Model file for the job. Use its own axes, mm. Face numbers are marked on the shaded views. A direction names the side the tool comes from. Give positions to 0.01 mm unless a question says otherwise; leave off trailing zeros. Loops run counter-clockwise (first coordinate to the right, second up) from the corner with the lowest first, then second, coordinate; pieces in that order, holes last. Notation, with made-up numbers: M 60.5,43 L 85.5,43 A9 cw 85.5,47 Z; hole C 15,33.5 d8. An arc over 180 degrees is marked long. Answer in a Markdown table with one row per item.
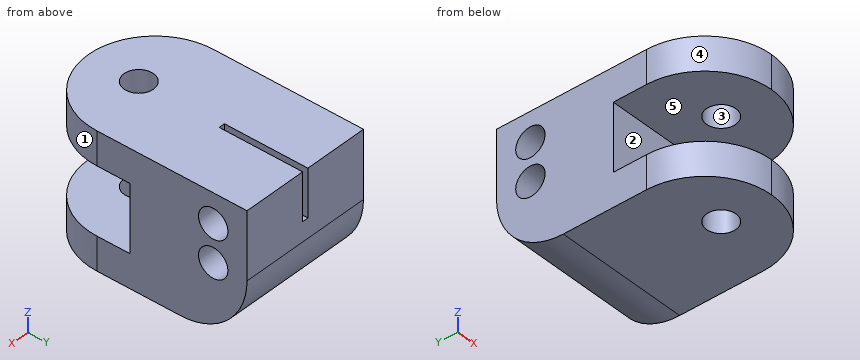
```python
from build123d import *

# Parameters (mm, degrees)
F0_W      = 10.16
F0_H      = 10.16
F1_DEPTH  = 10.16
F2_T      = -2.54
F3_W      = 10.16
F3_H      = 10.16
F4_DEPTH  = 6.35
F5_R      = 1.1176
F6_DEPTH  = 10.16
F7_R      = 1.1176
F8_DEPTH  = 10.16
F9_R      = 5.07999
F10_W     = 0.4572
F10_H     = 6.35
F11_DEPTH = 3.6068


# Not quite as in the source:
# - a fillet or chamfer is up to 0.001 mm smaller than in the source, because OpenCascade refuses the exact size


with BuildPart() as f1:
    # F0 (on Front) → F1 (new body)
    with BuildSketch(Plane.XZ):
        Rectangle(F0_W, F0_H)
    extrude(amount=F1_DEPTH)

    # F2
    f2_openings = [f1.faces().sort_by_distance(p)[0] for p in [
        (0, -10.16, 0),
        (5.08, -5.08, 0),
        (-5.08, -5.08, 0),
    ]]
    offset(amount=F2_T, openings=f2_openings)

    # F3 (on face) → F4 (join)
    with BuildSketch(Plane(origin=(0, 0, 0), x_dir=(-1, 0, 0), z_dir=(0, 1, 0))):
        Rectangle(F3_W, F3_H)
    extrude(amount=F4_DEPTH)

    # F5 (on face) → F6 (cut)
    with BuildSketch(Plane.YZ.offset(5.08)):
        with Locations((3.7731814664, 0)):
            Circle(F5_R)
        with Locations((3.7731814664, 2.838186454)):
            Circle(F5_R)
    extrude(amount=-F6_DEPTH, mode=Mode.SUBTRACT)

    # F7 (on face) → F8 (cut)
    with BuildSketch(Plane.XY.offset(5.08)):
        with Locations((0, -6.3200981603)):
            Circle(F7_R)
    extrude(amount=-F8_DEPTH, mode=Mode.SUBTRACT)

    # F9 (radius 5.08 in the source; OpenCascade refuses exactly that, so slightly less here)
    f9_edges = [f1.edges().sort_by_distance(p)[0] for p in [
        (5.08, -10.16, -3.81),
        (5.08, -10.16, 3.81),
        (-5.08, -10.16, 3.81),
        (-5.08, -10.16, -3.81),
        (0, 6.35, -5.08),
    ]]
    fillet(f9_edges, radius=F9_R)

    # F10 (on face) → F11 (cut)
    with BuildSketch(Plane.XY.offset(5.08)):
        with Locations((0, 3.175)):
            Rectangle(F10_W, F10_H)
    extrude(amount=-F11_DEPTH, mode=Mode.SUBTRACT)


solid = f1.part
```
(1) Which spindle directions (+Z, -Z, +X, -X, +Y, -Y) get a long thin tool onto all of the face, cutting with end or side? Do the marked faces 4 and 5. Say none if no direction does.
Established:
| item | result |
|---|---|
| face 4 | +Z, -Z, -X, -Y |
| face 5 | +X, -X, -Y |
(2) Saw through at C-C, the plane y = 3.5. Give the cut face in (x, z), and give its area (3 significant figures).
Established:
| item | result |
|---|---|
| outline | M -5.08,-4.56 L 5.08,-4.56 L 5.08,-1.08 L -5.08,-1.08 Z; M -5.08,1.08 L 5.08,1.08 L 5.08,1.75 L 0.23,1.75 L 0.23,1.47 L -0.23,1.47 L -0.23,1.75 L -5.08,1.75 Z; M -5.08,3.92 L -0.23,3.92 L -0.23,5.08 L -5.08,5.08 Z; M 0.23,3.92 L 5.08,3.92 L 5.08,5.08 L 0.23,5.08 Z |
| area | 53.3 mm2 |
(3) Saw through at A-A, the plane z = 3.5. Count the separate pieces of the cut face and the enclosed holes in it, and give its area (3 significant figures).
Established:
| item | result |
|---|---|
| separate pieces | 3 |
| enclosed holes | 1 |
| area | 132 mm2 |
(4) Saw through at B-B, the plane x = 0.75. Give the cut face in (y, z), and give its area (3 significant figures).
Established:
| item | result |
|---|---|
| outline | M -10.1,-5.08 L -7.15,-5.08 L -7.15,-2.54 L -10.1,-2.54 Z; M -10.1,2.54 L -7.15,2.54 L -7.15,5.08 L -10.1,5.08 Z; M -5.49,-5.08 L 1.27,-5.08 A5.08 ccw 6.35,0 L 6.35,5.08 L -5.49,5.08 L -5.49,2.54 L -2.54,2.54 L -2.54,-2.54 L -5.49,-2.54 Z; hole C 3.77,0 d2.24; hole C 3.77,2.84 d2.24 |
| area | 107 mm2 |
(5) Mould opens along X. For the marked faces 1, 2 and 3 say: pulls with the +X half, pulls with the -X half, needs draft (parallel to the pull), parting line crosses it, or undercut.
Established:
| item | result |
|---|---|
| face 1 | pulls with the +X half |
| face 2 | needs draft |
| face 3 | undercut |
(6) Flat gauge pins, fed straight in: P1, Ø5.5, axis at x = 2.5, z = -1, coming from the -Y side; P2, Ø2, axis at y = 3.77, z = 0, coming from the +X side; P3, Ø1.5, axis at x = 2, z = -4, coming from the +Y side; P4, Ø3, axis at x = 3.5, z = -4, coming from the +Y side. Where does each tip first touch, or does it go through?
Established:
| item | result |
|---|---|
| P1 | stops at y = -10.16 |
| P2 | passes through |
| P3 | stops at y = 5.17 |
| P4 | stops at y = 5.69 |
(7) Saw through at D-D, the plane x = -3.5. Give the cut face in (y, z), and give its area (3 significant figures).
Established:
| item | result |
|---|---|
| outline | M -8.76,-5.08 L 1.27,-5.08 A5.08 ccw 6.35,0 L 6.35,5.08 L -8.76,5.08 L -8.76,2.54 L -2.54,2.54 L -2.54,-2.54 L -8.76,-2.54 Z; hole C 3.77,0 d2.24; hole C 3.77,2.84 d2.24 |
| area | 109 mm2 |
(8) Wall check: L1, parallel to Z at x = 0.5, y = -9.5; L2, parallel to Z at x = -2.75, y = 3; L3, parallel to Y at x = 0, z = 3.75. Give the ranges that are in metal, low to high.
Established:
| item | result |
|---|---|
| L1 | z = -5.08 to -2.54, 2.54 to 5.08 |
| L2 | z = -4.78 to -0.81, 0.81 to 2.03, 3.65 to 5.08 |
| L3 | y = -10.16 to -7.44, -5.2 to 0 |
